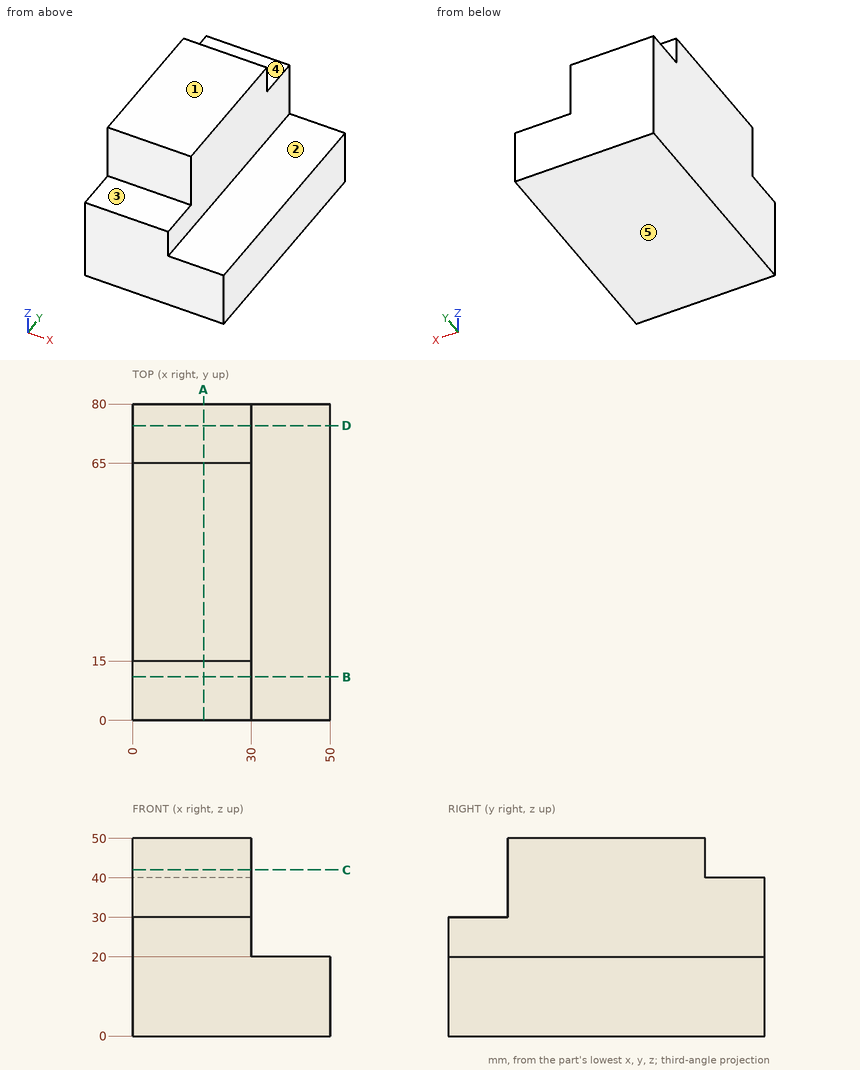
Check sheet for the drawn part. Datum: minimum x, y, z corner. Units: mm. A direction names the side the tool comes from. Coordinates: 2 decimals unless noted, no trailing zeros. Order: outer loops, then holes, each group sorted by start corner. A loop starts at its lowest first (then second) coordinate and runs counter-clockwise, first axis right, second up. Notation, with made-up numbers: M 44,63 L 77,63 A22 cw 77,75 Z; hole C -9,6.5 d1. An arc over 180 degrees is marked long. One line per item, written item: value. Start each with the question number.
Item 1: Gauge pin test, flat ends, axial feed: pin 1 (9 mm diameter, centred on y = 59.5, z = 31.5, fed in from +X); pin 2 (8 mm diameter, centred on x = 12.5, z = 46.5, fed in from +Y); pin 3 (1.5 mm diameter, centred on x = 45, y = 26.5, fed in from +Z). Record the tip position at first contact, or that the pin passes through.
Item 2: Sectioned sample at A-A (x = 18). Enter the section's corners in (y, z), then the cut area to 3 significant figures.
Item 3: Sectioned sample at D-D (y = 74.5). Enter the section's corners in (x, z).
Item 4: Sectioned sample at C-C (z = 42). Enter the section's corners in (x, y).
Item 5: Scan lines: probe 1 along X at (y, z) = (40, 23); probe 2 along Z at (x, y) = (45, 67.5); probe 3 along Z at (x, y) = (3, 68). Record each from-to range of solid material in increasing order.
Item 6: Access from +Z, -Z, +X, -X, +Y, -Y to the whole of each face (thin tool, end or side, straight path). Record for the marked faces 1, 2, 3, 4 and 5.
Item 7: Sectioned sample at B-B (y = 11). Enter the section's corners in (x, z).
Conclusion:
1. pin 1: stops at x = 30
1. pin 2: stops at y = 65
1. pin 3: stops at z = 20
2. outline: M 0,0 L 80,0 L 80,40 L 65,40 L 65,50 L 15,50 L 15,30 L 0,30 Z
2. area: 3,550 mm^2
3. outline: M 0,0 L 50,0 L 50,20 L 30,20 L 30,40 L 0,40 Z
4. outline: M 0,15 L 30,15 L 30,65 L 0,65 Z
5. probe 1: x = 0 to 30
5. probe 2: z = 0 to 20
5. probe 3: z = 0 to 40
6. face 1: +Z, +X, -X, +Y, -Y
6. face 2: +Z, +X, +Y, -Y
6. face 3: +Z, +X, -X, -Y
6. face 4: +Z, +X, -X, +Y
6. face 5: -Z, +X, -X, +Y, -Y
7. outline: M 0,0 L 50,0 L 50,20 L 30,20 L 30,30 L 0,30 Z
